```python
from build123d import *

# Parameters (mm, degrees)
F1_DEPTH = 44
F2_R     = 10
F4_DEPTH = 50.9


with BuildPart() as f1:
    # F0 (on Front) → F1 (new body)
    with BuildSketch(Plane.XZ):
        with BuildLine():
            Line((18, 7.333334), (-22, 7.333334))
            Line((-22, 7.333334), (-22, -25.666667))
            Line((-22, -25.666667), (33, -25.666667))
            Line((33, -25.666667), (33, -7.666666))
            ThreePointArc((33, -7.666666), (43.606602, 17.939935), (18, 7.333334))
        make_face()
    extrude(amount=F1_DEPTH)

    # F2
    f2_edges = [f1.edges().sort_by_distance(p)[0] for p in [
        (5.5, -44, -25.666667),
        (33, -44, -16.666667),
        (-22, -44, -9.166667),
    ]]
    fillet(f2_edges, radius=F2_R)

    # F3 (on face) → F4 (cut)
    with BuildSketch(Plane(origin=(0, 0, -25.666667), x_dir=(1, 0, 0), z_dir=(0, 0, -1))):
        with BuildLine():
            Line((15.25307, 21.926958), (-4.803377, 21.926958))
            Line((-4.803377, 21.926958), (-4.803377, 9.747743))
            Line((-4.803377, 9.747743), (20.25307, 9.747743))
            Line((20.25307, 9.747743), (20.25307, 16.926958))
            ThreePointArc((20.25307, 16.926958), (18.788604, 20.462492), (15.25307, 21.926958))
        make_face()
    extrude(amount=-F4_DEPTH, mode=Mode.SUBTRACT)


solid = f1.part
```
The listing builds one solid part. Answer for the finished solid, in the listing's coordinates (mm). A direction names the side the tool comes from. Give positions to 0.01 mm unless a question says otherwise; leave off trailing zeros. Write each loop counter-clockwise with the first axis right and the second up, starting at its lowest first coordinate (ties: lowest second). Pieces come first, ordered by that corner, then holes. Notation, with made-up numbers: (-13, 73) - (0, 73) arc R4 cw to (0, 80) - close; hole circle Ø6 at (-25, 85.25). An arc over 180 degrees is marked (long way). Use one line per item in the form item = value. Start each with the question number.
1) Find section A-A on y = -13. Determine the outline of the cut face in (x, z), plus the area to 3 significant figures.
2) The mould has two halves that part along Y. Classify faces 1 (the face through (5, -9, -25.667)), 2 (the face through (5, -21.927, -9)), 3 (the face through (5.89, -40.99, -22.82)), 4 (the face through (20.253, -13, -5)): pulls with the +Y half, pulls with the -Y half, needs draft (parallel to the pull), parting line crosses it, or undercut.
3) Find section D-D on x = 26.5. Determine the outline of the cut face in (y, z).
4) Flat-ended cylindrical pins translate along their axes: pin 1 Ø3 at (x, z) = (-14.5, -15.5) entering from -Y; pin 2 Ø20 at (y, z) = (-18, -20) entering from +X; pin 3 Ø1 at (y, z) = (-32.5, 9) entering from +X. Find the tip coordinate at first contact, or state that the pin passes through.
5) A tool of negligible diameter and unlimited length cuts with its end or side. For faces 5 (the face through (18.83, -20.42, -5.5)), 6 (the face through (-6, -22, 7.333)), 7 (the face through (33, -17, -17)), from which of +Z, -Z, +X, -X, +Y, -Y can it reach the whole face along a straight path? Write none if from no direction.
6) Find section C-C on z = -17. Determine the outline of the cut face in (x, y).
7) Consider line 1 along Y through (x, z) = (1.5, -0.5); line 2 along X through (y, z) = (-23.5, -14.5); line 3 along Z through (x, y) = (6, -9.5). Determine where each line is inside the solid, lowest interval first. Write a range as from..to.
8) Find section B-B on x = 0. Determine the outline of the cut face in (y, z), plus the area to 3 significant figures.
Geometry results:
q1.outline = (-22, -25.67) - (-4.8, -25.67) - (-4.8, 7.33) - (-22, 7.33) - close; (20.25, -25.67) - (33, -25.67) - (33, -7.67) arc R15 ccw (long way) to (20.25, 15.24) - close
q1.area = 1,510 mm2
q2.face_1 = needs draft
q2.face_2 = undercut
q2.face_3 = pulls with the -Y half
q2.face_4 = undercut
q3.outline = (-44, -6.19) - (-43.37, -6.19) - (-43.37, -19.17) arc R10 ccw to (-34, -25.67) - (0, -25.67) - (0, 20.85) - (-44, 20.85) - close
q4.pin_1 = -43.95
q4.pin_2 = 33
q4.pin_3 = 47.95
q5.face_5 = +Z, -Z
q5.face_6 = +Z, -X, +Y, -Y
q5.face_7 = -Z, +X, +Y, -Y
q6.outline = (-22, -34) arc R10 ccw to (-13.33, -43.91) - (24.33, -43.91) arc R10 ccw to (33, -34) - (33, 0) - (-22, 0) - close; hole (-4.8, -21.93) - (15.25, -21.93) arc R5 ccw to (20.25, -16.93) - (20.25, -9.75) - (-4.8, -9.75) - close
q7.line_1 = -44..-21.93, -9.75..0
q7.line_2 = -22..33
q7.line_3 = -25.67..7.33
q8.outline = (-44, -15.67) arc R10 ccw to (-34, -25.67) - (-21.93, -25.67) - (-21.93, 7.33) - (-44, 7.33) - close; (-9.75, -25.67) - (0, -25.67) - (0, 7.33) - (-9.75, 7.33) - close
q8.area = 1,030 mm2
